Design review of the part built by this model. Coordinates are the model's own, in mm. Face numbers are marked on the shaded views. A direction names the side the tool comes from. Coordinates: 2 decimals unless noted, no trailing zeros. Write each loop counter-clockwise with the first axis right and the second up, starting at its lowest first coordinate (ties: lowest second). Pieces come first, ordered by that corner, then holes.
Q1. For pin 1 Ø0.6 at (y, z) = (2.5, -4.5) entering from -X; pin 2 Ø1 at (x, y) = (5, 4) entering from +Z; pin 3 Ø1.5 at (x, z) = (-1, 1.5) entering from -Y; pin 4 Ø2 at (x, y) = (-3.5, 3) entering from +Z, all flat-tipped, find the tip position at first contact; note any pin that passes through.
Q2. Take a section at C-C, the plane y = 1.4. Write out the cut boundary in (x, z).
Q3. Take a section at D-D, the plane x = -3.25. Write out the cut boundary in (y, z).
Q4. For the marked faces 1, 2 and 3, list the 3-axis set-ups (+Z, -Z, +X, -X, +Y, -Y) from which the entire face can be reached by the end or side of a thin tool; tool diameter is ignored.
Q5. For L1, parallel to X at y = 3.5, z = -2.05; L2, parallel to Z at x = -3.75, y = 1.75; L3, parallel to Z at x = -3, y = 2.45, list the stretches that pass through material, from the lowest coordinate up.
Q6. Take a section at B-B, the plane x = 1.25. Write out the cut boundary in (y, z), plus the area to 3 significant figures.
Q7. Take a section at A-A, the plane z = -2.05. Write out the cut boundary in (x, y).
Q8. The part is to be moulded in two halves that separate along Z. For the marked faces 4, 5 and 6, say which applies: released by +Z, released by -Z, zero draft, split by the parting line, or undercut.
from build123d import *

# Parameters (mm, degrees)
SKETCH_1_W      = 12.8
SKETCH_1_H      = 6.5
SKETCH_1_R      = 1
EXTRUDE_1_DEPTH = 5.8
SKETCH_2_W      = 0.8
SKETCH_2_H      = 0.5
EXTRUDE_2_DEPTH = 3.5
SKETCH_4_W      = 0.142011972
SKETCH_4_H      = 5.5
EXTRUDE_4_DEPTH = 0.5
EXTRUDE_5_DEPTH = 5.5


with BuildPart() as part:
    # 草图1 → 凸台-拉伸1 (new body)
    with BuildSketch(Plane(origin=(0, 0, 0), x_dir=(1, 0, 0), z_dir=(0, 1, 0))):
        Rectangle(SKETCH_1_W, SKETCH_1_H)
        with Locations(Location((-3.25, 2.05, 0), (0, 0, 270))):
            Circle(SKETCH_1_R, mode=Mode.SUBTRACT)
        with Locations(Location((3.25, 2.05, 0), (0, 0, 90))):
            Circle(SKETCH_1_R, mode=Mode.SUBTRACT)
    extrude(amount=EXTRUDE_1_DEPTH)

    # 草图2 → 凸台-拉伸2 (add)
    with BuildSketch(Plane(origin=(0, 0, -3.25), x_dir=(-1, 0, 0), z_dir=(0, 0, -1))):
        with Locations((0, 2.801277115)):
            Rectangle(SKETCH_2_W, SKETCH_2_H)
        with Locations((5.08, 2.801277115)):
            Rectangle(SKETCH_2_W, SKETCH_2_H)
        with Locations((-5.08, 2.801277115)):
            Rectangle(SKETCH_2_W, SKETCH_2_H)
    extrude(amount=EXTRUDE_2_DEPTH)

    # 草图4 → 凸台-拉伸4 (add)
    with BuildSketch(Plane.XY.offset(3.25)):
        with Locations((-5.9, 2.9)):
            Rectangle(SKETCH_4_W, SKETCH_4_H)
    extrude(amount=EXTRUDE_4_DEPTH)

    # 草图6 → 凸台-拉伸5 (add)
    with BuildSketch(Plane.XZ.offset(-0.15)):
        Polygon((-5.828994014, 3.75), (-5.828994014, 3.5), (7.03115002, 4.998700306), (7.03115002, 5.248700306), align=None)
    extrude(amount=-EXTRUDE_5_DEPTH)


solid = part.part
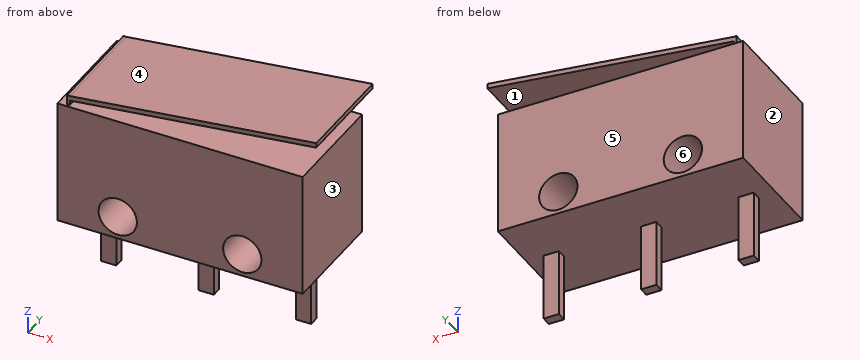
Responses:
1. pin 1: stops at x = -5.48
1. pin 2: stops at z = 5.07
1. pin 3: stops at y = 0
1. pin 4: stops at z = 4.14
2. outline: (-6.4, -3.25) - (6.4, -3.25) - (6.4, 3.25) - (-5.83, 3.25) - (-5.83, 3.5) - (7.03, 5) - (7.03, 5.25) - (-5.83, 3.75) - (-5.97, 3.75) - (-5.97, 3.25) - (-6.4, 3.25) - close; hole circle Ø2 at (-3.25, -2.05); hole circle Ø2 at (3.25, -2.05)
3. outline: (0, -3.25) - (5.8, -3.25) - (5.8, -3.05) - (0, -3.05) - close; (0, -1.05) - (5.8, -1.05) - (5.8, 3.25) - (0, 3.25) - close; (0.15, 3.8) - (5.65, 3.8) - (5.65, 4.05) - (0.15, 4.05) - close
4. face 1: +X, +Y, -Y
4. face 2: +Z, -Z, -X, +Y, -Y
4. face 3: -Z, +X, +Y, -Y
5. L1: x = -6.4 to -4.25, -2.25 to 2.25, 4.25 to 6.4
5. L2: z = -3.25 to -2.92, -1.18 to 3.25, 3.74 to 3.99
5. L3: z = -3.25 to -3.02, -1.08 to 3.25, 3.83 to 4.08
6. outline: (0, -3.25) - (5.8, -3.25) - (5.8, 3.25) - (0, 3.25) - close; (0.15, 4.32) - (5.65, 4.32) - (5.65, 4.57) - (0.15, 4.57) - close
6. area: 39.1 mm2
7. outline: (-6.4, 0) - (-4.25, 0) - (-4.25, 5.8) - (-6.4, 5.8) - close; (-2.25, 0) - (2.25, 0) - (2.25, 5.8) - (-2.25, 5.8) - close; (4.25, 0) - (6.4, 0) - (6.4, 5.8) - (4.25, 5.8) - close
8. face 4: released by +Z
8. face 5: zero draft
8. face 6: undercut
